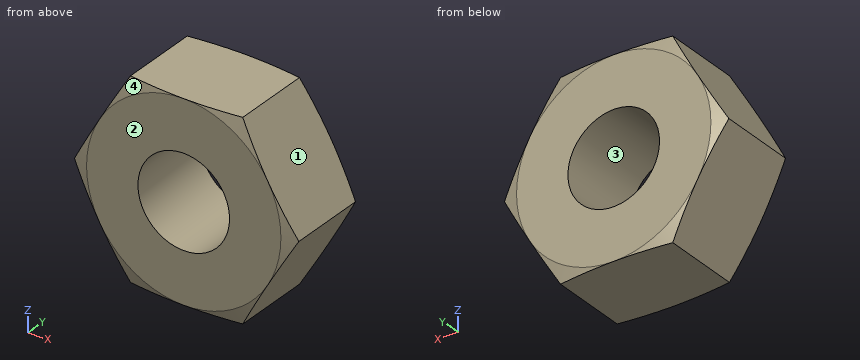
from build123d import *

# Parameters (mm, degrees)
EXTRUDE_1_DEPTH    = 3.1
HOLE_WIZARD_M4_1_D = 3.3


with BuildPart() as part:
    # 草图1 → 凸台-拉伸1 (new body)
    with BuildSketch(Plane(origin=(0, 0, 0), x_dir=(1, 0, 0), z_dir=(0, 1, 0))):
        Polygon((4.041451884, 0), (2.020725942, 3.5), (-2.020725942, 3.5), (-4.041451884, 0), (-2.020725942, -3.5), (2.020725942, -3.5), align=None)
    extrude(amount=EXTRUDE_1_DEPTH)

    # M4 螺纹孔1 (through all)
    with Locations(Plane(origin=(0, 3.1, 0), x_dir=(1, 0, 0), z_dir=(0, 1, 0))):
        with Locations((0, 0)):
            Hole(HOLE_WIZARD_M4_1_D / 2)

    # 草图5 → 切除-旋转1 (revolve, cut)
    with BuildSketch(Plane(origin=(0, 0, 0), x_dir=(0, 0, -1), z_dir=(1, 0, 0))):
        Polygon((-3.5, 0), (-4.387126804, 0.237704911), (-4.387126804, -0.855779568), align=None)
        Polygon((-4.387126804, 3.955779568), (-3.5, 3.1), (-4.387126804, 2.862295089), align=None)
    revolve(axis=Axis((0, 0, 0), (0, -1, 0)), mode=Mode.SUBTRACT)


solid = part.part
Here's how the part is built. I have some questions about the finished solid (model axes, mm). Face numbers are marked on the shaded views. Round coordinates to 2 decimals unless told otherwise and drop trailing zeros. Loops run counter-clockwise (first coordinate to the right, second up) from the corner with the lowest first, then second, coordinate; pieces in that order, holes last. Notation, with made-up numbers: (35.5, 82) - (54.5, 82) arc R29 ccw to (54.5, 119) - close; hole circle Ø4 at (14, -18). An arc over 180 degrees is marked (long way). One line per question, with ' | ' between items. Start each with the question number.
Q1. We'd pull the mould along X, two halves only. Please class the marked faces 1, 2, 3 and 4: +X half, -X half, draft (parallel to the pull), parting line (faces both ways), or undercut.
Q2. Please list where these lines run through material, in increasing order: line 1 (Z direction, x = 0, y = 2.35); line 2 (Z direction, x = -1, y = 2.7); line 3 (X direction, y = 2.8, z = 0.75). Write a range as [from, to].
Q3. Will these pins go through, and if not, where does the flat tip stop? pin 1 (1 mm diameter, centred on y = 1.5, z = -2, fed in from -X); pin 2 (1 mm diameter, centred on y = 1, z = 2.5, fed in from +X).
Q4. I want a section at A-A (y = 2.8). Write out the boundary of the cut face in (x, z), then the cut area to 3 significant figures.
Response values:
1) face 1: +X half | face 2: draft | face 3: undercut | face 4: -X half
2) line 1: z = [-3.5, -1.65], [1.65, 3.5] | line 2: z = [-3.5, -1.31], [1.31, 3.5] | line 3: x = [-3.61, -1.47], [1.47, 3.61]
3) pin 1: stops at x = -3.18 | pin 2: stops at x = 2.89
4) outline: (-4.04, 0) - (-2.02, -3.5) - (2.02, -3.5) - (4.04, 0) - (2.02, 3.5) - (-2.02, 3.5) - close; hole circle Ø3.3 at (0, 0) | area: 33.9 mm²
